from build123d import *

# Parameters (mm, degrees)
F0_W         = 50
F0_H         = 40
F1_DEPTH     = 2.5
F7_R         = 4
F7_R_2       = 2.05
F10_DEPTH    = 8
F11_SIZE2    = 39.99999
F11_SIZE     = 6.99999
F6_R         = 2.05
F12_DEPTH    = 46.3
F13_R        = 2.05
F14_DEPTH    = 68.7
F15_T4_DEPTH = 50
F15_S5_R     = 4
F15_T6_DEPTH = 35
F15_S7_R     = 4
F15_T8_DEPTH = 35


# Not quite as in the source:
# - a fillet or chamfer that OpenCascade refuses, or shapes differently, is made with other operations: its cross-section is extruded or revolved along the edge and cut away or added
# - a fillet or chamfer is up to 0.001 mm smaller than in the source, because OpenCascade refuses the exact size


with BuildPart() as f1:
    # F0 (on Top) → F1 (new body)
    with BuildSketch(Plane.XY):
        Rectangle(F0_W, F0_H)
    extrude(amount=F1_DEPTH)

    # F7 (on offset) → F8 (join, up to the last surface of F1)
    with BuildSketch(Plane(origin=(-11.6521931986, 0, 20.1821906397), x_dir=(0.8660254038, 0, 0.5), z_dir=(0.5, 0, -0.8660254038))):
        with Locations((-6.8889131071, 0.075317279)):
            Circle(F7_R)
        with Locations((-6.8889131071, 0.075317279)):
            Circle(F7_R_2, mode=Mode.SUBTRACT)
    extrude(until=Until.LAST)

    # F9: F1 across plane


with BuildPart() as f1_1:
    add(f1.part)
    add(f1.part.mirror(Plane.YZ))

    # F0 (on Top) → F10 (join)
    with BuildSketch(Plane.XY):
        Rectangle(F0_W, F0_H)
    extrude(amount=-F10_DEPTH)

    # F11 (size 7 and 40 in the source; OpenCascade refuses exactly that, so slightly less here)
    f11_edges = [f1_1.edges().sort_by_distance(p)[0] for p in [
        (0, 20, -8),
    ]]
    f11_side = f1_1.faces().sort_by_distance((0, 20, -2.75))[0]
    chamfer(f11_edges, length=F11_SIZE, length2=F11_SIZE2, reference=f11_side)

    # F6 (on offset) → F12 (cut)
    with BuildSketch(Plane(origin=(-11.6521931986, 0, 20.1821906397), x_dir=(0.8660254038, 0, 0.5), z_dir=(0.5, 0, -0.8660254038))):
        with Locations((-6.8571413867, 0.094557312)):
            Circle(F6_R)
    extrude(amount=F12_DEPTH, mode=Mode.SUBTRACT)

    # F13 (on offset) → F14 (cut)
    with BuildSketch(Plane(origin=(11.6521931986, 0, 20.1821906397), x_dir=(0.8660254038, 0, -0.5), z_dir=(0.5, 0, 0.8660254038))):
        with Locations((6.8889131072, -0.075317279)):
            Circle(F13_R)
    extrude(amount=-F14_DEPTH, mode=Mode.SUBTRACT)

    # F15: chamfer of 7 x 40 on 1 edges, made by hand


with BuildPart() as f15_tool2:
    # F15_s3 → F15_t4 (new body)
    with BuildSketch(Plane.YZ.offset(-25)):
        with BuildLine():
            Line((21.5760487474, 2.7758085308), (-21.5760487474, -4.7758085308))
            Line((-21.5760487474, -4.7758085308), (-22.3760487474, -4.7758085308))
            ThreePointArc((-22.3760487474, -4.7758085308), (-20.8, -1.1379042654), (-20.8, 2.5))
            Line((-20.8, 2.5), (-20, 3.3))
            ThreePointArc((-20, 3.3), (0.7880243737, 3.3), (21.5760487474, 3.5758085308))
            Line((21.5760487474, 3.5758085308), (21.5760487474, 2.7758085308))
        make_face()
    extrude(amount=F15_T4_DEPTH)

    # F15_s5 → F15_t6 (cut, symmetric)
    with BuildSketch(Plane(origin=(0.25, 0, -0.4330127019), x_dir=(0, 1, 0), z_dir=(-0.5, 0, 0.8660254038))):
        with Locations((-0.075317279, 6.8889131071)):
            Circle(F15_S5_R)
    extrude(amount=F15_T6_DEPTH, both=True, mode=Mode.SUBTRACT)

    # F15_s7 → F15_t8 (cut, symmetric)
    with BuildSketch(Plane(origin=(-0.25, 0, -0.4330127019), x_dir=(0, 1, 0), z_dir=(0.5, 0, 0.8660254038))):
        with Locations((-0.075317279, -6.8889131071)):
            Circle(F15_S7_R)
    extrude(amount=F15_T8_DEPTH, both=True, mode=Mode.SUBTRACT)


with BuildPart() as f1_2:
    add(f1_1.part)

    # F15_t1: cut F15_tool2
    add(f15_tool2.part, mode=Mode.SUBTRACT)


solid = f1_2.part
The listing builds one solid part. Answer for the finished solid, in the listing's coordinates (mm). Coordinates: 2 decimals unless noted, no trailing zeros. Order: outer loops, then holes, each group sorted by start corner. A loop starts at its lowest first (then second) coordinate and runs counter-clockwise, first axis right, second up. Notation, with made-up numbers: (78.25, -4) -> (103.25, -4) arc R10 cw to (103.25, 8) -> close; hole circle Ø1 at (-2.5, -22.5). An arc over 180 degrees is marked (long way). Answer in a Markdown table with one row per item. Add a question column.
Item 1: Find section D-D (y = 12.5). Write down the section's boundary in (x, z).
Item 2: Determine the mould class of faces 1 (the face through (0, 0, -1)), 2 (the face through (-16.127, 1.646, 17.599)), 3 (the face through (0, -20, -6)), 4 (the face through (-15, 0.9, 8.6)) for opening direction Y: +Y half, -Y half, draft (parallel to the pull), parting line (faces both ways), or undercut.
Item 3: Find the intervals of material crossed by L1, parallel to Y at x = 14, z = 10; L2, parallel to Z at x = 12, y = -3 (3 decimals); L3, parallel to Z at x = 19.5, y = 6.5, in increasing order. Write a range as from..to.
Item 4: Find section C-C (z = -6). Write down the section's boundary in (x, y).
Item 5: Find section B-B (z = 8). State how many separate pieces and enclosed holes the cut face has, then the cut area to 3 significant figures.
Item 6: Find section A-A (y = -1). Write down the section's boundary in (x, z) (3 decimals).
Item 7: Each of these flat-tipped pins is pushed along its axis until it touches: P1, Ø2, axis at x = 7.5, y = 15.5, coming from the +Z side; P2, Ø10, axis at x = -5, y = -5, coming from the +Z side; P3, Ø4, axis at x = 9.5, y = 11, coming from the +Z side (3 decimals). Where does it stop, or does it pass through?
Result set:
| question | item | result |
|---|---|---|
| 1 | outline | (-25, -2.31) -> (25, -2.31) -> (25, 1.19) -> (-25, 1.19) -> close |
| 2 | face 1 | undercut |
| 2 | face 2 | draft |
| 2 | face 3 | -Y half |
| 2 | face 4 | undercut |
| 3 | L1 | y = -4.07..-2.11, 1.96..3.92 |
| 3 | L2 | z = -5.025..-1.525, 1.549..12.464 |
| 3 | L3 | z = -3.36..0.14 |
| 4 | outline | (-25, -20) -> (25, -20) -> (25, -8.57) -> (-25, -8.57) -> close |
| 5 | separate pieces | 2 |
| 5 | enclosed holes | 2 |
| 5 | area | 85.4 mm² |
| 6 | outline | (-25, -4.675) -> (-7.343, -4.675) -> (-11.485, 2.5) -> (-11.511, 2.5) -> (-19.203, 15.823) -> (-20.988, 14.792) -> (-11.77, -1.175) -> (-25, -1.175) -> close; (-15.998, 17.673) -> (-3.095, -4.675) -> (3.143, -4.675) -> (16.034, 17.653) -> (14.248, 18.684) -> (2.783, -1.175) -> (-2.783, -1.175) -> (-14.248, 18.684) -> close; (7.368, -4.675) -> (25, -4.675) -> (25, -1.175) -> (11.77, -1.175) -> (20.988, 14.792) -> (19.203, 15.823) -> close |
| 7 | P1 | stops at z = 1.89 |
| 7 | P2 | stops at z = 8.84 |
| 7 | P3 | stops at z = 1.275 |
